Study the drawing (mm; zero at the part's minimum x, y, z) and answer. Give positions to 0.01 mm unless a question says otherwise; leave off trailing zeros. Use a Markdown table: item, result. Add a question column.
Item 1: A cutting plane is placed at A-A on y = 19.05. Count the separate pieces of the cut face and the enclosed holes in it.
Item 2: Consider probe 1 along Y at (x, z) = (19.05, 1.1); probe 2 along X at (y, z) = (31.5, 0.75); probe 3 along X at (y, z) = (30.5, 1.4) (1 decimal). Determine where each line is inside the solid, lowest interval first. Write a range as [from, to].
Item 3: The mould has two halves that part along Y. Classify the marked faces 1, 2 and 3: pulls with the +Y half, pulls with the -Y half, needs draft (parallel to the pull), parting line crosses it, or undercut.
Item 4: Given P1, Ø11.5, axis at x = 17.5, y = 20.5, coming from the +Z side (3 decimals); P2, Ø1, axis at y = 7.5, z = 0.5, coming from the +X side, each flat-ended and moving along its own axis, determine where each tip first touches the part or whether it passes through.
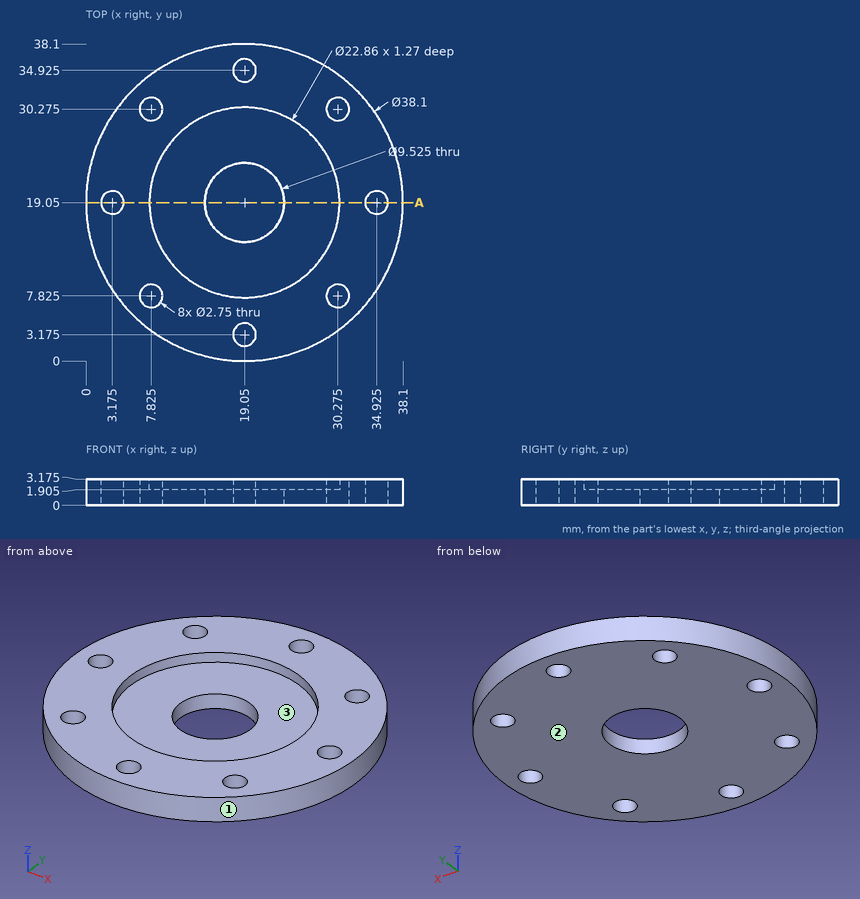
Filled in:
| question | item | result |
|---|---|---|
| 1 | separate pieces | 4 |
| 1 | enclosed holes | 0 |
| 2 | probe 1 | [0, 1.8], [4.55, 14.29], [23.81, 33.55], [36.3, 38.1] |
| 2 | probe 2 | [4.63, 7.2], [8.45, 29.65], [30.9, 33.47] |
| 2 | probe 3 | [3.8, 6.5], [9.2, 28.9], [31.6, 34.3] |
| 3 | face 1 | parting line crosses it |
| 3 | face 2 | needs draft |
| 3 | face 3 | undercut |
| 4 | P1 | z = 1.905 |
| 4 | P2 | x = 34.57 |
